The model under review builds one solid part; all positions refer to its coordinate system, in mm. Round coordinates to 2 decimals unless told otherwise and drop trailing zeros. Order: outer loops, then holes, each group sorted by start corner. A loop starts at its lowest first (then second) coordinate and runs counter-clockwise, first axis right, second up. Notation, with made-up numbers: M -32,27.25 L -6,27.25 A10 ccw -6,43.25 Z; hole C 55,30 d11. An arc over 180 degrees is marked long. Answer as a JSON object with one key per item and string values. Group by question number.
1. To check wall thickness, follow probe 1 along X at (y, z) = (-4.75, -3); probe 2 along Z at (x, y) = (-83, -5); probe 3 along Z at (x, y) = (-354, 9). State the ranges of each line that lie inside material, in increasing order. Write a range as [from, to].
2. Add section B-B on z = 0. State the section outline as (x, y) points.
3. Clearance check with flat-ended pins moving along their axes: P1, Ø20.5, axis at x = 128, z = -14, coming from the +Y side; P2, Ø6, axis at y = 1.5, z = -19, coming from the -X side; P3, Ø4, axis at y = -6, z = -8, coming from the +X side; P4, Ø12, axis at x = 143, z = -27, coming from the -Y side. State where each tip first meets the part, or that it passes through.
4. Add section C-C on y = -4.5. State the section outline as (x, z) points.
5. Add section A-A on x = 117.5. State the section outline as (y, z) points, and give its area (3 significant figures).
```python
from build123d import *

# Parameters (mm, degrees)
F1_DEPTH = 10
F3_DEPTH = 7.5


with BuildPart() as f1:
    # F0 (on Front) → F1 (new body, symmetric)
    with BuildSketch(Plane.XZ):
        with BuildLine():
            Line((394, 36.7), (-394, 36.7))
            ThreePointArc((-394, 36.7), (-430.7, 0), (-394, -36.7))
            Line((-394, -36.7), (394, -36.7))
            ThreePointArc((394, -36.7), (430.7, 0), (394, 36.7))
        make_face()
        with BuildLine():
            Line((394, -34.5), (-394, -34.5))
            ThreePointArc((-394, -34.5), (-428.5, 0), (-394, 34.5))
            Line((-394, 34.5), (394, 34.5))
            ThreePointArc((394, 34.5), (428.5, 0), (394, -34.5))
        make_face(mode=Mode.SUBTRACT)
    extrude(amount=F1_DEPTH, both=True)

    # F2 (on Front) → F3 (join, symmetric)
    with BuildSketch(Plane.XZ):
        with BuildLine():
            Line((394, 34.5), (-394, 34.5))
            ThreePointArc((-394, 34.5), (-428.5, 0), (-394, -34.5))
            Line((-394, -34.5), (394, -34.5))
            ThreePointArc((394, -34.5), (428.5, 0), (394, 34.5))
        make_face()
        with BuildLine():
            ThreePointArc((-394, -31.1), (-425.1, 0), (-394, 31.1))
            Line((-394, 31.1), (394, 31.1))
            ThreePointArc((394, 31.1), (425.1, 0), (394, -31.1))
            Line((394, -31.1), (-394, -31.1))
        make_face(mode=Mode.SUBTRACT)
    extrude(amount=F3_DEPTH, both=True)


solid = f1.part
```
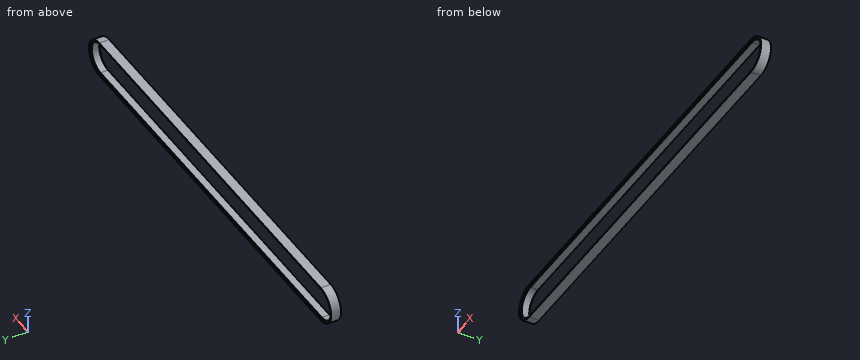
Recorded:
{
 "1": {"probe 1": "x = [-430.58, -424.95], [424.95, 430.58]", "probe 2": "z = [-36.7, -31.1], [31.1, 36.7]", "probe 3": "z = [-36.7, -34.5], [34.5, 36.7]"},
 "2": {"outline": "M -430.7,-10 L -428.5,-10 L -428.5,-7.5 L -425.1,-7.5 L -425.1,7.5 L -428.5,7.5 L -428.5,10 L -430.7,10 Z; M 425.1,-7.5 L 428.5,-7.5 L 428.5,-10 L 430.7,-10 L 430.7,10 L 428.5,10 L 428.5,7.5 L 425.1,7.5 Z"},
 "3": {"P1": "passes through", "P2": "stops at x = -427.03", "P3": "stops at x = 430.21", "P4": "stops at y = -7.5"},
 "4": {"outline": "M -394,-36.7 L 394,-36.7 A36.7 ccw 394,36.7 L -394,36.7 A36.7 ccw Z; hole M -394,-31.1 L 394,-31.1 A31.1 ccw 394,31.1 L -394,31.1 A31.1 ccw Z"},
 "5": {"outline": "M -10,-36.7 L 10,-36.7 L 10,-34.5 L 7.5,-34.5 L 7.5,-31.1 L -7.5,-31.1 L -7.5,-34.5 L -10,-34.5 Z; M -10,34.5 L -7.5,34.5 L -7.5,31.1 L 7.5,31.1 L 7.5,34.5 L 10,34.5 L 10,36.7 L -10,36.7 Z", "area": "190 mm²"}
}
